Job drawing, mm, ordinate dimensions from the low corner. One solid piece. Coordinates: 2 decimals unless noted, no trailing zeros. Loops run counter-clockwise (first coordinate to the right, second up) from the corner with the lowest first, then second, coordinate; pieces in that order, holes last. Notation, with made-up numbers: (-0.5, 45) -> (52.5, 45) arc R11 ccw to (52.5, 53) -> close; hole circle Ø5 at (75, 60.5). An arc over 180 degrees is marked (long way). Answer as CSV lines item,"result". Start each with the question number.
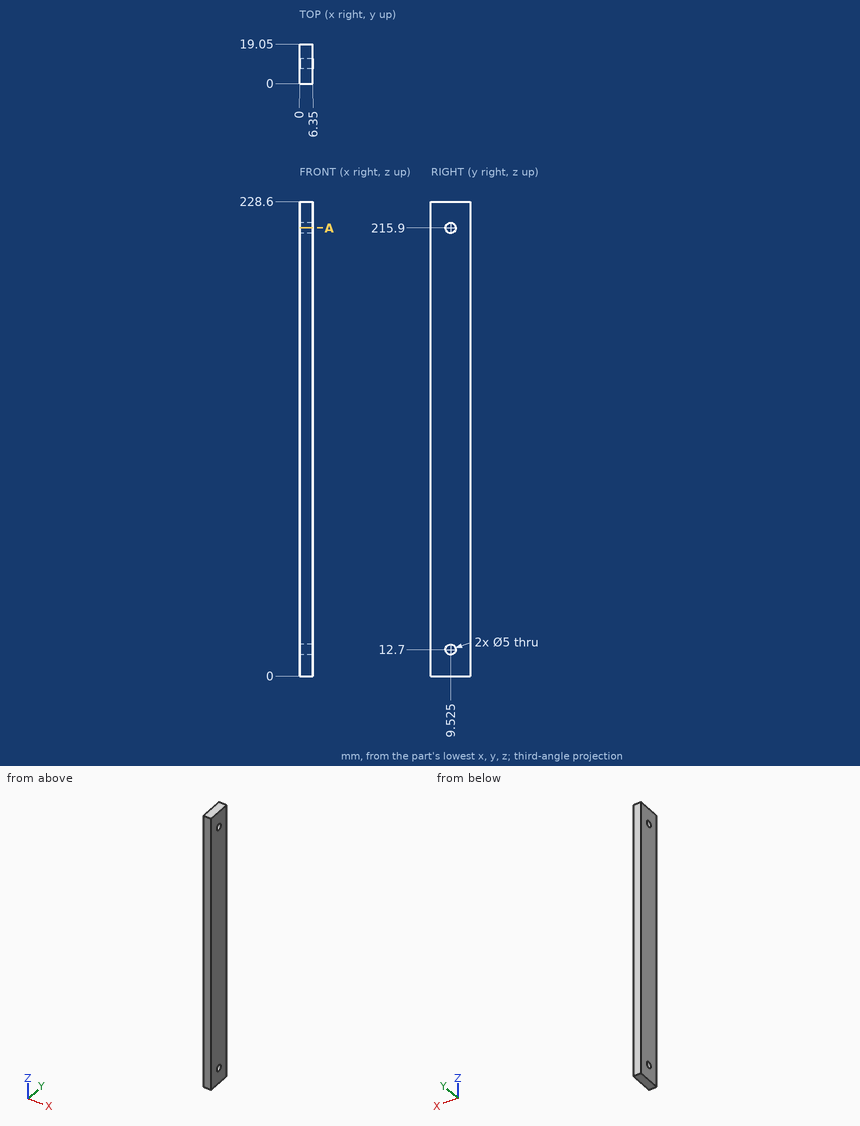
Item 1: Wall check: probe 1 along Y at (x, z) = (2.5, 12.7) (3 decimals); probe 2 along Z at (x, y) = (0.75, 10); probe 3 along Z at (x, y) = (2, 11.5). Give the ranges that are in metal, low to high.
Item 2: Flat gauge pin, fed straight in: pin 1 Ø3 at (y, z) = (9.525, 12.7) entering from +X. Where does the tip first touch, or does it go through?
Item 3: Saw through at A-A (z = 215.9). Write the cut outline in (x, y) (3 decimals), plus the area to 3 significant figures.
Geometry check:
1,probe 1,"0 to 7.025, 12.025 to 19.05"
1,probe 2,"0 to 10.25, 15.15 to 213.45, 218.35 to 228.6"
1,probe 3,"0 to 11.17, 14.23 to 214.37, 217.43 to 228.6"
2,pin 1,"through"
3,outline,"(0, 0) -> (6.35, 0) -> (6.35, 7.025) -> (0, 7.025) -> close; (0, 12.025) -> (6.35, 12.025) -> (6.35, 19.05) -> (0, 19.05) -> close"
3,area,"89.2 mm2"
